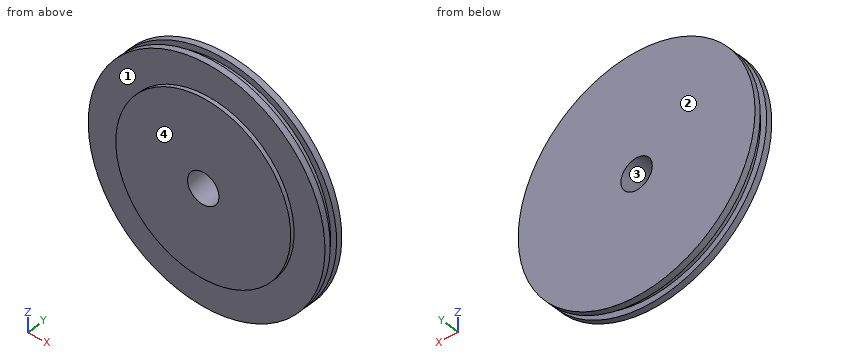
```python
from build123d import *

# Parameters (mm, degrees)
SKETCH6_R                   = 4.1021
F_5_16_CLOSE_FIT_HOLE_DEPTH = 45.063579292
BOSS_EXTRUDE1_START         = 1.016
SKETCH7_R                   = 22.86
SKETCH7_R_2                 = 4.1021
BOSS_EXTRUDE1_DEPTH         = 1.016


with BuildPart() as part:
    # Sketch1 → Revolve1 (revolve)
    with BuildSketch(Plane(origin=(0, 0, 0), x_dir=(0, 0, -1), z_dir=(1, 0, 0))):
        Polygon((0, 0), (0, -5.08), (-30.9499, -5.08), (-30.9499, -3.5052), (-29.3878, -3.5052), (-29.3878, -1.5748), (-30.9499, -1.5748), (-30.9499, 0), align=None)
    revolve(axis=Axis((0, 0, 0), (0, -1, 0)))

    # Sketch6 → 5/16 Close Fit hole (cut, through all)
    with BuildSketch(Plane.XZ.offset(5.08)):
        with Locations(Location((0, 0, 0), (0, 0, 270))):
            Circle(SKETCH6_R)
    extrude(amount=-F_5_16_CLOSE_FIT_HOLE_DEPTH, mode=Mode.SUBTRACT)

    # Sketch7 → Boss-Extrude1 (add)
    with BuildSketch(Plane.XZ.offset(5.08).offset(BOSS_EXTRUDE1_START)):
        with Locations(Location((0, 0, 0), (0, 0, 270))):
            Circle(SKETCH7_R)
        with Locations(Location((0, 0, 0), (0, 0, 270))):
            Circle(SKETCH7_R_2, mode=Mode.SUBTRACT)
    extrude(amount=-BOSS_EXTRUDE1_DEPTH)


solid = part.part
```
Can you work these out from the model? Positions are in its coordinate system, mm. Face numbers are marked on the shaded views. A direction names the side the tool comes from. Coordinates: 2 decimals unless noted, no trailing zeros. Write each loop counter-clockwise with the first axis right and the second up, starting at its lowest first coordinate (ties: lowest second). Pieces come first, ordered by that corner, then holes. Notation, with made-up numbers: M 8,19 L 28,19 A34 ccw 28,55 Z; hole C 60,74.25 d5. An arc over 180 degrees is marked long. Write item = value, one per line. Start each with the question number.
Q1. If we section it at A-A, the plane x = 0: Write out the boundary of the cut face in (y, z).
Q2. On a 3-axis mill with a long thin cutter (end or side, diameter ignored), from which of +Z, -Z, +X, -X, +Y, -Y can I reach the whole of each face in a straight line? I mean the marked faces 1 and 2. Say none if no direction works.
Q3. If we section it at D-D, the plane x = -9.5: Write out the boundary of the cut face in (y, z).
Q4. If we section it at C-C, the plane z = -6.5: Write out the boundary of the cut face in (x, y).
Q5. I'm going to push flat-ended pins straight in: pin 1 (3 mm diameter, centred on y = -0.5, z = -15.5, fed in from +X); pin 2 (1.5 mm diameter, centred on y = -3.5, z = -22, fed in from +X); pin 3 (2 mm diameter, centred on x = 14, z = 19.5, fed in from -Y). Where does each tip first touch, or does it pass through?
Q6. If we section it at B-B, the plane z = 0: Write out the boundary of the cut face in (x, y).
Q7. Thinking about a two-plate mould opening in Z: for the marked faces 3 and 4, which applies, released by +Z, released by -Z, zero draft, split by the parting line, or undercut?
Q8. If I drill on L1, parallel to X at y = -2.75, z = 0; L2, parallel to Y at x = 5.5, z = 26; L3, parallel to Z at x = 2.5, y = -4.5, over which ranges is the centre line in solid material (lowest first)? Write a range as [from, to].
Check sheet entries:
q1.outline = M -6.1,-22.86 L -5.08,-22.86 L -5.08,-30.95 L -3.51,-30.95 L -3.51,-29.39 L -1.57,-29.39 L -1.57,-30.95 L 0,-30.95 L 0,-4.1 L -6.1,-4.1 Z; M -6.1,4.1 L 0,4.1 L 0,30.95 L -1.57,30.95 L -1.57,29.39 L -3.51,29.39 L -3.51,30.95 L -5.08,30.95 L -5.08,22.86 L -6.1,22.86 Z
q2.face_1 = -Y
q2.face_2 = +Z, -Z, +X, -X, +Y
q3.outline = M -6.1,-20.79 L -5.08,-20.79 L -5.08,-29.46 L -3.51,-29.46 L -3.51,-27.81 L -1.57,-27.81 L -1.57,-29.46 L 0,-29.46 L 0,29.46 L -1.57,29.46 L -1.57,27.81 L -3.51,27.81 L -3.51,29.46 L -5.08,29.46 L -5.08,20.79 L -6.1,20.79 Z
q4.outline = M -30.26,-5.08 L -21.92,-5.08 L -21.92,-6.1 L 21.92,-6.1 L 21.92,-5.08 L 30.26,-5.08 L 30.26,-3.51 L 28.66,-3.51 L 28.66,-1.57 L 30.26,-1.57 L 30.26,0 L -30.26,0 L -30.26,-1.57 L -28.66,-1.57 L -28.66,-3.51 L -30.26,-3.51 Z
q5.pin_1 = 27.6
q5.pin_2 = 22.5
q5.pin_3 = -5.08
q6.outline = M -30.95,-5.08 L -22.86,-5.08 L -22.86,-6.1 L -4.1,-6.1 L -4.1,0 L -30.95,0 L -30.95,-1.57 L -29.39,-1.57 L -29.39,-3.51 L -30.95,-3.51 Z; M 4.1,-6.1 L 22.86,-6.1 L 22.86,-5.08 L 30.95,-5.08 L 30.95,-3.51 L 29.39,-3.51 L 29.39,-1.57 L 30.95,-1.57 L 30.95,0 L 4.1,0 Z
q7.face_3 = undercut
q7.face_4 = zero draft
q8.L1 = [-29.39, -4.1], [4.1, 29.39]
q8.L2 = [-5.08, 0]
q8.L3 = [-30.85, -3.25], [3.25, 30.85]
